Verification items for the finished model (mm, model axes). Coordinates: 2 decimals unless noted, no trailing zeros.
Q1. Go/stop test with flat-tipped pins: P1, Ø0.5, axis at y = 13.5, z = 679, coming from the -X side; P2, Ø0.8, axis at x = -13.5, z = 1342.5, coming from the -Y side; P3, Ø2, axis at y = -0.5, z = 1403.5, coming from the -X side; P4, Ø1, axis at x = 3.5, y = -8, coming from the -Z side. Record where each tip stops, or that it passes through.
Q2. Sectioned sample at A-A (z = 426). Count the separate pieces of the cut face and the enclosed holes in it, then the cut area to 3 significant figures.
Q3. Material ranges on probe 1 along Y at (x, z) = (9.75, 137); probe 2 along X at (y, z) = (10, 1425); probe 3 along X at (y, z) = (11, 1615) (3 decimals), recorded low to high.
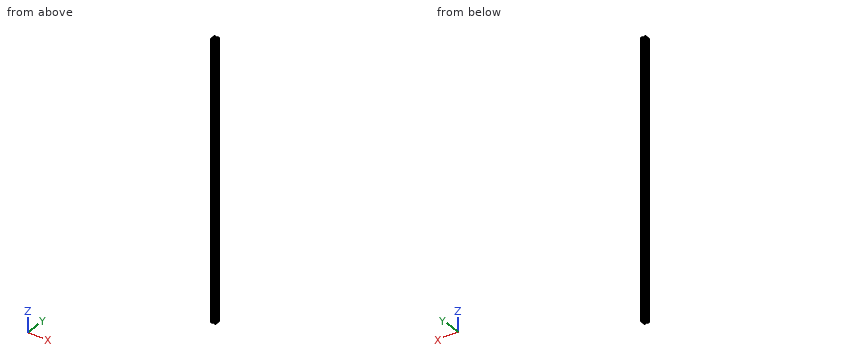
```python
from build123d import *

# Parameters (mm, degrees)
BOSS_EXTRUDE1_DEPTH     = 1828.8
CUT_EXTRUDE1_DEPTH      = 1
CUT_EXTRUDE1_DEPTH_BACK = 1829.8


with BuildPart() as part:
    # Sketch4 → Boss-Extrude1 (new body)
    with BuildSketch(Plane.XY):
        with BuildLine():
            Line((0, -5.45), (0.655464476, -6))
            Line((0.655464476, -6), (4.504469158, -6))
            Line((4.504469158, -6), (8.25, -9.745530842))
            Line((8.25, -9.745530842), (8.25, -12.885))
            Line((8.25, -12.885), (4, -12.885))
            Line((4, -12.885), (4, -14.45))
            Line((4, -14.45), (4.55, -14.45))
            Line((4.55, -14.45), (4.55, -15))
            Line((4.55, -15), (12.885, -15))
            ThreePointArc((12.885, -15), (14.380530842, -14.380530842), (15, -12.885))
            Line((15, -12.885), (15, -4.55))
            Line((15, -4.55), (14.45, -4.55))
            Line((14.45, -4.55), (14.45, -4))
            Line((14.45, -4), (12.885, -4))
            Line((12.885, -4), (12.885, -8.25))
            Line((12.885, -8.25), (9.745530842, -8.25))
            Line((9.745530842, -8.25), (6, -4.504469158))
            Line((6, -4.504469158), (6, -0.655464476))
            Line((6, -0.655464476), (5.45, 0))
            Line((5.45, 0), (3.5, 0))
            ThreePointArc((3.5, 0), (3.371433308, -0.939913534), (2.995178599, -1.81077474))
            Line((2.995178599, -1.81077474), (4.675743591, -3.491339732))
            Line((4.675743591, -3.491339732), (3.491339732, -4.675743591))
            Line((3.491339732, -4.675743591), (1.81077474, -2.995178599))
            ThreePointArc((1.81077474, -2.995178599), (0.939913534, -3.371433308), (0, -3.5))
            Line((0, -3.5), (0, -5.45))
        make_face()
        with BuildLine():
            Line((9.375, -10.365), (9.375, -12.885))
            ThreePointArc((9.375, -12.885), (9.664964287, -13.585035713), (10.365, -13.875))
            Line((10.365, -13.875), (12.885, -13.875))
            ThreePointArc((12.885, -13.875), (13.585035713, -13.585035713), (13.875, -12.885))
            Line((13.875, -12.885), (13.875, -10.365))
            ThreePointArc((13.875, -10.365), (13.585035713, -9.664964287), (12.885, -9.375))
            Line((12.885, -9.375), (10.365, -9.375))
            ThreePointArc((10.365, -9.375), (9.664964287, -9.664964287), (9.375, -10.365))
        make_face(mode=Mode.SUBTRACT)
    extrude(amount=BOSS_EXTRUDE1_DEPTH)

    # Mirror1: part across plane


with BuildPart() as part_1:
    add(part.part)
    add(part.part.mirror(Plane(origin=(0, 0, 0), x_dir=(0, 0, 1), z_dir=(1, 0, 0))))

    # Mirror2: part across plane


with BuildPart() as part_2:
    add(part_1.part)
    add(part_1.part.mirror(Plane.ZX))

    # Sketch5 → Cut-Extrude1 (cut, two sides)
    with BuildSketch(Plane.XY.offset(1828.8)) as cut_extrude1_sk:
        Polygon((-5.675, 12.885), (-5.4, 13.16), (-5.125, 12.885), align=None)
    extrude(amount=CUT_EXTRUDE1_DEPTH, mode=Mode.SUBTRACT)
    extrude(cut_extrude1_sk.sketch, amount=-CUT_EXTRUDE1_DEPTH_BACK, mode=Mode.SUBTRACT)


solid = part_2.part
```
Geometry check:
1. P1: stops at x = -14.97
1. P2: stops at y = -14.99
1. P3: stops at x = -6
1. P4: passes through
2. separate pieces: 1
2. enclosed holes: 5
2. area: 295 mm2
3. probe 1: y = -15 to -13.66, -9.59 to -8.25, 8.25 to 9.59, 13.66 to 15
3. probe 2: x = -15 to -13.81, -9.44 to -8.25, 8.25 to 9.44, 13.81 to 15
3. probe 3: x = -15 to -13.875, -9.375 to -8.25, 8.25 to 9.375, 13.875 to 15
